Design review of the part built by this model. Coordinates are the model's own, in mm. Face numbers are marked on the shaded views. A direction names the side the tool comes from. Coordinates: 2 decimals unless noted, no trailing zeros. Loops run counter-clockwise (first coordinate to the right, second up) from the corner with the lowest first, then second, coordinate; pieces in that order, holes last. Notation, with made-up numbers: (-3, 47) - (54, 47) arc R18 ccw to (54, 55) - close; hole circle Ø2 at (68.25, 12). An arc over 180 degrees is marked (long way). Answer in a Markdown table with one row per item. Add a question column.
(1) We need section C-C, the plane y = 26. Write out the cut boundary in (x, z), plus the area to 3 significant figures.
(2) The part is to be moulded in two halves that separate along Z. For the marked faces 1, 2, 3 and 4, say which applies: released by +Z, released by -Z, zero draft, split by the parting line, or undercut.
(3) Clearance check with flat-ended pins moving along their axes: pin 1 (10 mm diameter, centred on x = -35.5, y = 35, fed in from -Z); pin 2 (4 mm diameter, centred on x = 35.5, z = 28, fed in from +Y); pin 3 (12 mm diameter, centred on y = 32.5, z = -9.5, fed in from -X). State where each tip first meets the part, or that it passes through.
(4) We need section B-B, the plane z = -8. Write out the cut boundary in (x, y), plus the area to 3 significant figures.
(5) To check wall thickness, follow L1, parallel to Y at x = 0, z = 22.5; L2, parallel to X at y = 45, z = -22.5; L3, parallel to Y at x = -47.5, z = 20. State the ranges of each line that lie inside material, in increasing order. Write a range as [from, to].
(6) We need section D-D, the plane z = 25. Write out the cut boundary in (x, y), plus the area to 3 significant figures.
(7) For the marked faces 5, 6, 7 and 8, list the 3-axis set-ups (+Z, -Z, +X, -X, +Y, -Y) from which the entire face can be reached by the end or side of a thin tool; tool diameter is ignored.
(8) We need section A-A, the plane y = 45. Write out the cut boundary in (x, z), plus the area to 3 significant figures.
from build123d import *

# Parameters (mm, degrees)
EXTRUDE_1_DEPTH          = 10
SKETCH_3_R               = 30
EXTRUDE_2_DEPTH          = 60
CUT_EXTRUDE_START        = -30
SKETCH_4_R               = 10
CUT_EXTRUDE_1_DEPTH      = 60
EXTRUDE_3_DEPTH          = 10
CUT_EXTRUDE_2_DEPTH      = 94.134165377
CUT_EXTRUDE_2_DEPTH_BACK = 94.134165377
SKETCH_8_R               = 20
RIB_2_REACH              = 95.134
SKETCH_9_WALL_W          = 210.033760752
SKETCH_9_WALL_H          = 10


with BuildPart() as part:
    # 草图2 → 凸台-拉伸1 (new body)
    with BuildSketch(Plane(origin=(0, 0, 0), x_dir=(1, 0, 0), z_dir=(0, 1, 0))):
        with BuildLine():
            Line((53.609446504, 5), (43.609446504, 5))
            ThreePointArc((43.609446504, 5), (38.609446504, 0), (43.609446504, -5))
            Line((43.609446504, -5), (53.609446504, -5))
            ThreePointArc((53.609446504, -5), (50.723980057, -18.056871313), (44.709873121, -30))
            Line((44.709873121, -30), (-44.709873121, -30))
            ThreePointArc((-44.709873121, -30), (-50.723980057, -18.056871313), (-53.609446504, -5))
            Line((-53.609446504, -5), (-43.609446504, -5))
            ThreePointArc((-43.609446504, -5), (-38.609446504, 0), (-43.609446504, 5))
            Line((-43.609446504, 5), (-53.609446504, 5))
            ThreePointArc((-53.609446504, 5), (-50.723980057, 18.056871313), (-44.709873121, 30))
            Line((-44.709873121, 30), (44.709873121, 30))
            ThreePointArc((44.709873121, 30), (50.723980057, 18.056871313), (53.609446504, 5))
        make_face()
    extrude(amount=EXTRUDE_1_DEPTH)

    # 草图3 → 凸台-拉伸2 (add)
    with BuildSketch(Plane(origin=(0, 10, 0), x_dir=(1, 0, 0), z_dir=(0, 1, 0))):
        with Locations(Location((0, 0, 0), (0, 0, 270))):
            Circle(SKETCH_3_R)
    extrude(amount=EXTRUDE_2_DEPTH)

    # 草图4 → 切除-拉伸1 (cut)
    with BuildSketch(Plane.XY.offset(CUT_EXTRUDE_START)):
        with Locations(Location((0, 45, 0), (0, 0, 90))):
            Circle(SKETCH_4_R)
    extrude(amount=CUT_EXTRUDE_1_DEPTH, mode=Mode.SUBTRACT)

    # 草图7 → 凸台-拉伸3 (add)
    with BuildSketch(Plane(origin=(0, 10, 0), x_dir=(1, 0, 0), z_dir=(0, 1, 0))):
        with BuildLine():
            Line((-48.915465391, -22.5), (-19.843134833, -22.5))
            ThreePointArc((-19.843134833, -22.5), (-30, 0), (-19.843134833, 22.5))
            Line((-19.843134833, 22.5), (-48.915465391, 22.5))
            ThreePointArc((-48.915465391, 22.5), (-52.003864181, 13.948866071), (-53.609446504, 5))
            Line((-53.609446504, 5), (-43.609446504, 5))
            ThreePointArc((-43.609446504, 5), (-38.609446504, 0), (-43.609446504, -5))
            Line((-43.609446504, -5), (-53.609446504, -5))
            ThreePointArc((-53.609446504, -5), (-52.003864181, -13.948866071), (-48.915465391, -22.5))
        make_face()
        with BuildLine():
            Line((19.843134833, -22.5), (48.915465391, -22.5))
            ThreePointArc((48.915465391, -22.5), (52.003864181, -13.948866071), (53.609446504, -5))
            Line((53.609446504, -5), (43.609446504, -5))
            ThreePointArc((43.609446504, -5), (38.609446504, 0), (43.609446504, 5))
            Line((43.609446504, 5), (53.609446504, 5))
            ThreePointArc((53.609446504, 5), (52.003864181, 13.948866071), (48.915465391, 22.5))
            Line((48.915465391, 22.5), (19.843134833, 22.5))
            ThreePointArc((19.843134833, 22.5), (30, 0), (19.843134833, -22.5))
        make_face()
    extrude(amount=EXTRUDE_3_DEPTH)

    # 草图8 → 切除-拉伸2 (cut, two sides: drawn at the far end of the back side and taken through both)
    with BuildSketch(Plane(origin=(0, 70, 0), x_dir=(1, 0, 0), z_dir=(0, 1, 0)).offset(-CUT_EXTRUDE_2_DEPTH_BACK)):
        with Locations(Location((0, 0, 0), (0, 0, 270))):
            Circle(SKETCH_8_R)
    extrude(amount=CUT_EXTRUDE_2_DEPTH + CUT_EXTRUDE_2_DEPTH_BACK, mode=Mode.SUBTRACT)

    # 草图9 wall → 筋2 (add, up to next)
    with BuildSketch(Plane(origin=(34.316023147, 30, 0), x_dir=(0.394517672004, -0.918888353651, 0), z_dir=(0.918888353651, 0.394517672004, 0)), mode=Mode.PRIVATE) as rib_2_sk1:
        Rectangle(SKETCH_9_WALL_W, SKETCH_9_WALL_H)
    rib_2_tool1 = extrude(rib_2_sk1.sketch, amount=-RIB_2_REACH, mode=Mode.PRIVATE) - part.part
    rib_2 = rib_2_tool1.solids().sort_by_distance((34.316023147, 30, 0))[0]
    add(rib_2)

    # 镜向1: 筋2 across plane
    add(rib_2.mirror(Plane(origin=(0, 0, 0), x_dir=(0, 0, 1), z_dir=(1, 0, 0))))


solid = part.part
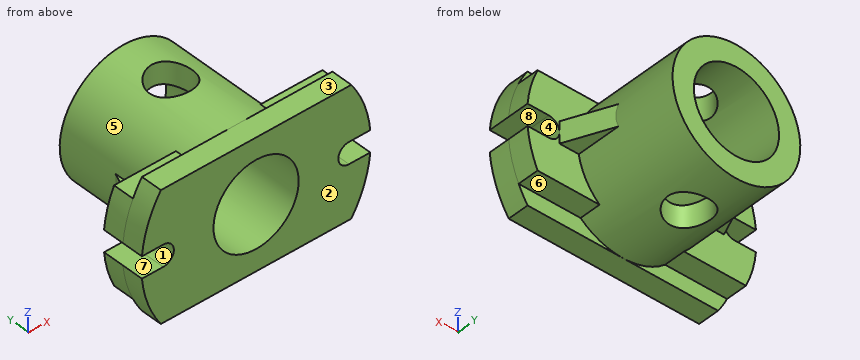
Responses:
| question | item | result |
|---|---|---|
| 1 | outline | (-36.03, -5) - (-29.58, -5) arc R30 ccw to (29.58, -5) - (36.03, -5) - (36.03, 5) - (29.58, 5) arc R30 ccw to (-29.58, 5) - (-36.03, 5) - close; hole circle Ø40 at (0, 0) |
| 1 | area | 1,690 mm2 |
| 2 | face 1 | undercut |
| 2 | face 2 | zero draft |
| 2 | face 3 | released by +Z |
| 2 | face 4 | undercut |
| 3 | pin 1 | stops at z = -5 |
| 3 | pin 2 | stops at y = 10 |
| 3 | pin 3 | stops at x = -34.95 |
| 4 | outline | (-53.24, 0) - (-18.33, 0) - (-18.33, 70) - (-28.91, 70) - (-28.91, 20) - (-53.24, 20) - close; (18.33, 0) - (53.24, 0) - (53.24, 20) - (28.91, 20) - (28.91, 70) - (18.33, 70) - close |
| 4 | area | 2,450 mm2 |
| 5 | L1 | y = [0, 35], [55, 70] |
| 5 | L2 | x = [-19.84, -10], [10, 19.84] |
| 5 | L3 | y = [0, 20] |
| 6 | outline | (-47.69, 0) - (47.69, 0) - (47.69, 10) - (16.58, 10) - (16.58, 70) - (-16.58, 70) - (-16.58, 10) - (-47.69, 10) - close; hole circle Ø20 at (0, 45) |
| 6 | area | 2,630 mm2 |
| 7 | face 5 | +Y |
| 7 | face 6 | -Z, +X, +Y |
| 7 | face 7 | -X, +Y, -Y |
| 7 | face 8 | +X, +Y, -Y |
| 8 | outline | (-10, -28.28) - (-10, -17.32) arc R20 cw to (-10, 17.32) - (-10, 28.28) arc R30 ccw to start; (10, -28.28) arc R30 ccw to (10, 28.28) - (10, 17.32) arc R20 cw to (10, -17.32) - close |
| 8 | area | 1,160 mm2 |
